For this review, use the dimensioned drawing (mm, ordinates from the lowest corner) and the shaded views. Round coordinates to 2 decimals unless told otherwise and drop trailing zeros. Loops run counter-clockwise (first coordinate to the right, second up) from the corner with the lowest first, then second, coordinate; pieces in that order, holes last.
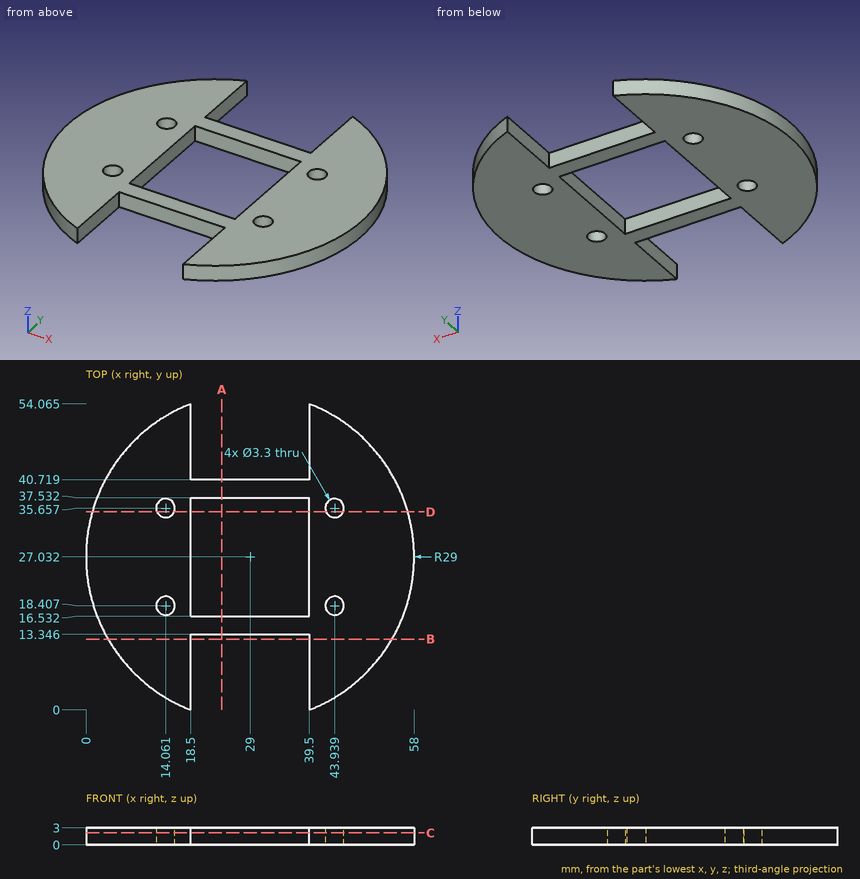
(1) Add section B-B (y = 12.5). Give the boundary of the cut face in (x, z).
(2) Add section C-C (z = 2.1). Give the number of separate pieces and of enclosed holes in the cut face, plus the area to 3 significant figures.
(3) Insertion check: pin 1 Ø1.5 at (y, z) = (14, 1) entering from -X; pin 2 Ø1.5 at (x, z) = (27, 1) entering from -Y; pin 3 Ø1.5 at (y, z) = (49.5, 1) entering from -X. Each pin has a flat end and moves straight along its axis. Give the tip position at first contact, or say it passes through.
(4) Add section D-D (y = 35). Give the boundary of the cut face in (x, z) (1 decimal).
(5) For L1, parallel to Y at x = 37, z = 0.25; L2, parallel to Y at x = 44.5, z = 1.9 (1 decimal); L3, parallel to Y at x = 13, z = 0.55 (1 decimal), list the stretches that pass through material, from the lowest coordinate up.
(6) Add section A-A (x = 24). Give the boundary of the cut face in (y, z).
Outcome:
1. outline: (3.9, 0) - (18.5, 0) - (18.5, 3) - (3.9, 3) - close; (39.5, 0) - (54.1, 0) - (54.1, 3) - (39.5, 3) - close
2. separate pieces: 1
2. enclosed holes: 5
2. area: 1,550 mm2
3. pin 1: stops at x = 2.73
3. pin 2: stops at y = 13.35
3. pin 3: stops at x = 9.78
4. outline: (1.1, 0) - (12.5, 0) - (12.5, 3) - (1.1, 3) - close; (15.6, 0) - (18.5, 0) - (18.5, 3) - (15.6, 3) - close; (39.5, 0) - (42.4, 0) - (42.4, 3) - (39.5, 3) - close; (45.5, 0) - (56.9, 0) - (56.9, 3) - (45.5, 3) - close
5. L1: y = 13.35 to 16.53, 37.53 to 40.72
5. L2: y = 2.5 to 16.9, 20 to 34.1, 37.2 to 51.5
5. L3: y = 2.8 to 17.1, 19.7 to 34.4, 36.9 to 51.2
6. outline: (13.35, 0) - (16.53, 0) - (16.53, 3) - (13.35, 3) - close; (37.53, 0) - (40.72, 0) - (40.72, 3) - (37.53, 3) - close
